Read the model definition and answer for the solid it produces. Units are mm, in the model's axes. A direction names the side the tool comes from. Give positions to 0.01 mm unless a question says otherwise; leave off trailing zeros. Order: outer loops, then holes, each group sorted by start corner. A loop starts at its lowest first (then second) coordinate and runs counter-clockwise, first axis right, second up. Notation, with made-up numbers: (78.5, -25) - (107.5, -25) arc R16 ccw to (107.5, -1) - close; hole circle Ø11 at (10.25, -6). An arc over 180 degrees is marked (long way). Answer as CSV lines item,"result". Start each with the question number.
from build123d import *

# Parameters (mm, degrees)
BOSS_EXTRU_1_DEPTH = 50


with BuildPart() as part:
    # Esquisse2 → Boss.-Extru.1 (new body)
    with BuildSketch(Plane.XY):
        with BuildLine():
            Line((-32.625, -8.920454545), (-32.625, 9.079545455))
            ThreePointArc((-32.625, 9.079545455), (-32.039213562, 10.493759017), (-30.625, 11.079545455))
            Line((-30.625, 11.079545455), (4.375, 11.079545455))
            ThreePointArc((4.375, 11.079545455), (5.789213562, 10.493759017), (6.375, 9.079545455))
            Line((6.375, 9.079545455), (6.375, -13.920454545))
            Line((6.375, -13.920454545), (1.875, -13.920454545))
            Line((1.875, -13.920454545), (1.875, 4.420454545))
            ThreePointArc((1.875, 4.420454545), (1.289213562, 5.834668108), (-0.125, 6.420454545))
            Line((-0.125, 6.420454545), (-26.125, 6.420454545))
            ThreePointArc((-26.125, 6.420454545), (-27.539213562, 5.834668108), (-28.125, 4.420454545))
            Line((-28.125, 4.420454545), (-28.125, -13.920454545))
            Line((-28.125, -13.920454545), (-32.625, -13.920454545))
            Line((-32.625, -13.920454545), (-32.625, -8.920454545))
        make_face()
    extrude(amount=BOSS_EXTRU_1_DEPTH)


solid = part.part
(1) Which of the six approach directions +Z, -Z, +X, -X, +Y, -Y give full straight-line access (tool end or side, diameter ignored) to faces 1 (the cylindrical face through (-32.055, 10.478, 24.65)), 2 (the flat face through (-28.125, -5, 25))?
(2) Section B-B, the plane z = 33.5 is taken. Write down the section's boundary in (x, y) (3 decimals).
(3) Straight lines are drawn through the part: line 1 (X direction, y = -2, z = 34) (3 decimals); line 2 (Y direction, x = -7.5, z = 45); line 3 (X direction, y = 4.75, z = 10) (3 decimals). For each, find the intervals that lie inside material, in ascending order. Write a range as [from, to].
(4) Section A-A, the plane y = -7.5 is taken. Write down the section's boundary in (x, z) (3 decimals), and give its area (3 significant figures).
(5) Determine the mould class of faces 3 (the flat face through (-30, -13.92, 25)), 4 (the cylindrical face through (1.305, 5.819, 24.65)), 5 (the cylindrical face through (-27.524, 5.85, 24.65)), 6 (the cylindrical face through (5.77, 10.51, 24.65)) for opening direction X: released by +X, released by -X, zero draft, split by the parting line, or undercut.
(6) Section C-C, the plane x = -19 is taken. Write down the section's boundary in (y, z).
(7) A flat-ended cylindrical pin translates along its axis: pin 1 Ø21 at (x, z) = (-9.5, 30.5) entering from -Y. Find the tip coordinate at first contact, or state that the pin passes through.
Checks:
1,face 1,"+Z, -Z, -X, +Y"
1,face 2,"+Z, -Z, -Y"
2,outline,"(-32.625, -13.92) - (-28.125, -13.92) - (-28.125, 4.42) arc R2 cw to (-26.125, 6.42) - (-0.125, 6.42) arc R2 cw to (1.875, 4.42) - (1.875, -13.92) - (6.375, -13.92) - (6.375, 9.08) arc R2 ccw to (4.375, 11.08) - (-30.625, 11.08) arc R2 ccw to (-32.625, 9.08) - close"
3,line 1,"x = [-32.625, -28.125], [1.875, 6.375]"
3,line 2,"y = [6.42, 11.08]"
3,line 3,"x = [-32.625, -28.098], [1.848, 6.375]"
4,outline,"(-32.625, 0) - (-28.125, 0) - (-28.125, 50) - (-32.625, 50) - close; (1.875, 0) - (6.375, 0) - (6.375, 50) - (1.875, 50) - close"
4,area,"450 mm²"
5,face 3,"zero draft"
5,face 4,"undercut"
5,face 5,"undercut"
5,face 6,"released by +X"
6,outline,"(6.42, 0) - (11.08, 0) - (11.08, 50) - (6.42, 50) - close"
7,pin 1,"stops at y = 6.07"
